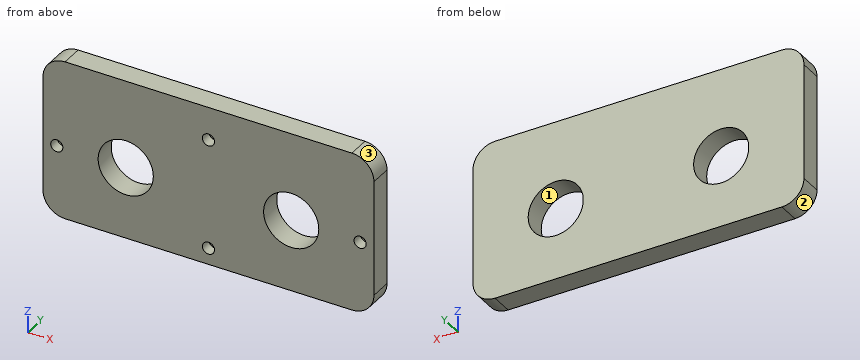
from build123d import *

# Parameters (mm, degrees)
F0_W     = 300
F0_H     = 160
F1_DEPTH = 10
F2_R     = 25
F3_DEPTH = 20.001
F4_R     = 5.5
F5_DEPTH = 10
F6_W     = 300
F6_H     = 15
F7_DEPTH = 20.001
F8_R     = 20


with BuildPart() as f1:
    # F0 (on Front) → F1 (new body, symmetric)
    with BuildSketch(Plane.XZ):
        Rectangle(F0_W, F0_H)
    extrude(amount=F1_DEPTH, both=True)

    # F2 (on face) → F3 (cut, through all)
    with BuildSketch(Plane.XZ.offset(10)):
        with Locations((-75, 0)):
            Circle(F2_R)
        with Locations((75, 0)):
            Circle(F2_R)
    extrude(amount=-F3_DEPTH, mode=Mode.SUBTRACT)

    # F4 (on face) → F5 (cut)
    with BuildSketch(Plane.XZ.offset(10)):
        with Locations((-137.5, 0)):
            Circle(F4_R)
        with Locations((0, 50)):
            Circle(F4_R)
        with Locations((137.5, 0)):
            Circle(F4_R)
        with Locations((0, -50)):
            Circle(F4_R)
    extrude(amount=-F5_DEPTH, mode=Mode.SUBTRACT)

    # F6 (on face) → F7 (cut, through all)
    with BuildSketch(Plane.XZ.offset(10)):
        with Locations((0, -72.5)):
            Rectangle(F6_W, F6_H)
    extrude(amount=-F7_DEPTH, mode=Mode.SUBTRACT)

    # F8
    f8_edges = [f1.edges().sort_by_distance(p)[0] for p in [
        (-150, 0, 80),
        (150, 0, 80),
        (-150, 0, -65),
        (150, 0, -65),
    ]]
    fillet(f8_edges, radius=F8_R)


solid = f1.part
Read the model definition and answer for the solid it produces. Units are mm, in the model's axes. Face numbers are marked on the shaded views. Give positions to 0.01 mm unless a question says otherwise; leave off trailing zeros. Write each loop counter-clockwise with the first axis right and the second up, starting at its lowest first coordinate (ties: lowest second). Pieces come first, ordered by that corner, then holes. Notation, with made-up numbers: (-2, 58.5) - (54, 58.5) arc R14 ccw to (54, 66.5) - close; hole circle Ø11 at (-23.75, 19.25). An arc over 180 degrees is marked (long way). Use CSV: the item, a comma, the result in double quotes. Start each with the question number.
Item 1: Consider line 1 (Z direction, x = 0, y = -2.75); line 2 (X direction, y = 1.25, z = -6.5); line 3 (X direction, y = -7.25, z = -16.5). Determine where each line is inside the solid, lowest interval first.
Item 2: Flat-ended cylindrical pins translate along their axes: P1, Ø3.5, axis at x = 1, z = -52.5, coming from the -Y side; P2, Ø1, axis at y = 4.5, z = -50.5, coming from the +X side. Find the tip coordinate at first contact, or state that the pin passes through.
Item 3: The part is cut by section C-C, the plane z = -19.5. Give the vertices of the cut face in (x, y), and give its area (3 significant figures).
Item 4: The mould has two halves that part along Z. Classify the marked faces 1, 2 and 3: pulls with the +Z half, pulls with the -Z half, needs draft (parallel to the pull), parting line crosses it, or undercut.
Item 5: The part is cut by section D-D, the plane x = 0. Give the vertices of the cut face in (y, z).
Item 6: The part is cut by section B-B, the plane x = -75. Give the vertices of the cut face in (y, z), and give its area (3 significant figures).
Item 7: The part is cut by section A-A, the plane y = -4.75. Give the vertices of the cut face in (x, z).
Taken from the geometry:
1,line 1,"-65 to -55.5, -44.5 to 44.5, 55.5 to 80"
1,line 2,"-150 to -99.14, -50.86 to 50.86, 99.14 to 150"
1,line 3,"-150 to -93.78, -56.22 to 56.22, 93.78 to 150"
2,P1,"y = 0"
2,P2,"x = 149.36"
3,outline,"(-150, -10) - (-90.64, -10) - (-90.64, 10) - (-150, 10) - close; (-59.36, -10) - (59.36, -10) - (59.36, 10) - (-59.36, 10) - close; (90.64, -10) - (150, -10) - (150, 10) - (90.64, 10) - close"
3,area,"4,750 mm2"
4,face 1,"undercut"
4,face 2,"pulls with the -Z half"
4,face 3,"pulls with the +Z half"
5,outline,"(-10, -65) - (10, -65) - (10, 80) - (-10, 80) - (-10, 55.5) - (0, 55.5) - (0, 44.5) - (-10, 44.5) - (-10, -44.5) - (0, -44.5) - (0, -55.5) - (-10, -55.5) - close"
6,outline,"(-10, -65) - (10, -65) - (10, -25) - (-10, -25) - close; (-10, 25) - (10, 25) - (10, 80) - (-10, 80) - close"
6,area,"1,900 mm2"
7,outline,"(-150, -45) arc R20 ccw to (-130, -65) - (130, -65) arc R20 ccw to (150, -45) - (150, 60) arc R20 ccw to (130, 80) - (-130, 80) arc R20 ccw to (-150, 60) - close; hole circle Ø11 at (-137.5, 0); hole circle Ø50 at (-75, 0); hole circle Ø11 at (0, -50); hole circle Ø11 at (0, 50); hole circle Ø50 at (75, 0); hole circle Ø11 at (137.5, 0)"
